Here's how the part is built. I have some questions about the finished solid (model axes, mm). A direction names the side the tool comes from. Round coordinates to 2 decimals unless told otherwise and drop trailing zeros. Write each loop counter-clockwise with the first axis right and the second up, starting at its lowest first coordinate (ties: lowest second). Pieces come first, ordered by that corner, then holes. Notation, with made-up numbers: (14, -28.5) -> (56, -28.5) arc R21 cw to (56, 10.5) -> close; hole circle Ø7 at (54, -9.75). An arc over 180 degrees is marked (long way). Answer as CSV lines item,"result".
Autodesk Inventor part; units mm, degrees
ref_plane "YZ Plane" through (0, 0, 0) normal (1, 0, 0) x (0, 1, 0)
ref_plane "XZ Plane" through (0, 0, 0) normal (0, 1, 0) x (-1, 0, 0)
ref_plane "XY Plane" through (0, 0, 0) normal (0, 0, 1) x (1, 0, 0)
sketch "Sketch1" plane through (0, 0, 0) normal (1, 0, 0) x (0, 1, 0)
  line L0 (0, 17.706) -> (3.1851, 17.706)
  line L1 (3.1851, 17.706) -> (3.1851, 5.3262)
  line L2 (3.1851, 5.3262) -> (5.2739, 5.3262)
  line L3 (5.2739, 5.3262) -> (5.2739, 2.5911)
  line L4 (5.2739, 2.5911) -> (3.8979, 2.5911)
  line L5 (3.8979, 2.5911) -> (3.8979, -0.2159)
  line L6 (3.8979, -0.2159) -> (5.2809, -0.2159)
  line L7 (5.2809, -0.2159) -> (5.2809, -3.3244)
  line L8 (5.2809, -3.3244) -> (3.8979, -3.3008)
  line L9 (3.8979, -3.3008) -> (3.8214, -7.7742)
  line L10 (3.8214, -7.7742) -> (0, -7.7742)
  line L11 (0, -7.7742) -> (0, 17.706)
  point P0 (0, 0)
revolve "Revolution1" add sketch "Sketch1" angle 360 about axis through (0, 0, -7.7742) along (0, 0, 1)
properties part number "simple_shaft"
1. If I drill on line 1 (Z direction, x = 3.5, y = 3.5); line 2 (X direction, y = -4.25, z = -2.25); line 3 (X direction, y = -3, z = 2.5), over which ranges is the centre line in solid material (lowest first)?
Numbers:
line 1,"z = -3.32 to -0.22, 2.59 to 5.33"
line 2,"x = -3.13 to 3.13"
line 3,"x = -2.49 to 2.49"
2. Suppose I cut it at B-B on z = 13.75. Please give me the cut outline in (x, y), and give its area (3 significant figures).
Numbers:
outline,"circle Ø6.37 at (0, 0)"
area,"31.9 mm^2"
3. On a 3-axis mill with a long thin cutter (end or side, diameter ignored), from which of +Z, -Z, +X, -X, +Y, -Y can I reach the whole of each face in a straight line? I mean faces 4 (the face through (3.16, -0.41, 11.43)), 5 (the face through (1.586, 5.037, -1.792)), 6 (the face through (2.3, -3.1, -5.5)). Say none if no direction works.
Numbers:
face 4,"+Z"
face 5,"+Z, -Z"
face 6,"-Z"
4. Suppose I cut it at A-A on z = -2.5. Please give me the cut outline in (x, y), and give its area (3 significant figures).
Numbers:
outline,"circle Ø10.56 at (0, 0)"
area,"87.6 mm^2"
5. For pin 1 Ø4 at (y, z) = (-2, 11.5) entering from +X; pin 2 Ø1 at (x, z) = (0, 7.5) entering from -Y; pin 3 Ø4 at (x, z) = (-1, 1) entering from -Y; pin 4 Ø6 at (y, z) = (-2.5, 6.5) entering from -X, each with a flat end and sliding along its axis, tell me the tip position at first contact or that it passes through.
Numbers:
pin 1,"stops at x = 3.19"
pin 2,"stops at y = -3.19"
pin 3,"stops at y = -5.28"
pin 4,"stops at x = -5.27"
6. If we mould it in two halves opening along Z, with no side actions, what happens to faces 1 (the face through (0, 0, -7.774)), 2 (the face through (0, 0, 17.706)), 3 (the face through (-3.805, -0.845, 1.168))? For each: released by +Z, released by -Z, zero draft, split by the parting line, or undercut.
Numbers:
face 1,"released by -Z"
face 2,"released by +Z"
face 3,"undercut"
